from build123d import *
from OCP.BRepFilletAPI import BRepFilletAPI_MakeChamfer

# Parameters (mm, degrees)
SKETCH1_W               = 120
SKETCH1_H               = 38
SKETCH1_W_2             = 41
SKETCH1_H_2             = 21
BOSS_EXTRUDE1_DEPTH     = 11
SKETCH2_R               = 1.3
CUT_EXTRUDE1_DEPTH      = 8
FILLET1_RADIUS          = 19
FILLET1_LENGTH          = 11
BOSS_EXTRUDE2_START     = 8
BOSS_EXTRUDE2_DEPTH     = 8
FILLET2_R               = 16
CUT_EXTRUDE2_DEPTH      = 66.741919656
CUT_EXTRUDE2_DEPTH_BACK = 66.741919656
BOSS_EXTRUDE3_START     = 8
BOSS_EXTRUDE3_OUTLINE_W = 32
BOSS_EXTRUDE3_OUTLINE_H = 8
BOSS_EXTRUDE3_DEPTH     = 49
SKETCH6_W               = 52
SKETCH6_H               = 38
BOSS_EXTRUDE4_DEPTH     = 8
CUT_EXTRUDE3_DEPTH      = 74.518705262
CUT_EXTRUDE3_DEPTH_BACK = 74.518705262
SKETCH7_W               = 31
SKETCH7_H               = 13
SKETCH8_W               = 13
SKETCH8_H               = 23
CUT_EXTRUDE4_DEPTH      = 8
BOSS_EXTRUDE5_START     = -2
SKETCH9_R               = 9
BOSS_EXTRUDE5_DEPTH     = 2
SKETCH10_R              = 6.5
CUT_EXTRUDE5_DEPTH      = 8
SKETCH12_W              = 5
SKETCH12_H              = 6
CUT_EXTRUDE6_DEPTH      = 20
CHAMFER1_SIZE           = 6
CHAMFER1_SIZE_2         = 20
FILLET3_R               = 8
FILLET4_R               = 6
FILLET5_R               = 6
FILLET6_R               = 2.5
SKETCH13_R              = 1.1
CUT_EXTRUDE7_DEPTH      = 8
CUT_EXTRUDE8_DEPTH      = 69.483574828
CUT_EXTRUDE8_DEPTH_BACK = 69.483574828
CUT_EXTRUDE9_DEPTH      = 66.741919805
CUT_EXTRUDE9_DEPTH_BACK = 66.741919805
SKETCH15_R              = 1.3
SKETCH16_R              = 1.1
BOSS_EXTRUDE6_DEPTH     = 8
SKETCH17_R              = 1
CUT_EXTRUDE10_DEPTH     = 7


# Read off the part's stored shape, not the designer's step: Boss-Extrude3
# Some blends are built 0.0001 mm under size
with BuildPart() as part:
    # Sketch1 → Boss-Extrude1 (new body)
    with BuildSketch(Plane.XY):
        Rectangle(SKETCH1_W, SKETCH1_H)
        with Locations((-24.5, 0)):
            Rectangle(SKETCH1_W_2, SKETCH1_H_2, mode=Mode.SUBTRACT)
    extrude(amount=BOSS_EXTRUDE1_DEPTH)

    # Sketch2 → Cut-Extrude1 (cut)
    with BuildSketch(Plane.XY.offset(1)):
        with Locations((0, 5)):
            Circle(SKETCH2_R)
        with Locations((-48, 5)):
            Circle(SKETCH2_R)
        with Locations((-48, -5)):
            Circle(SKETCH2_R)
        with Locations((0, -5)):
            Circle(SKETCH2_R)
    extrude(amount=CUT_EXTRUDE1_DEPTH, mode=Mode.SUBTRACT)

    # Fillet1: full round fillet: the end face becomes a half cylinder, R = half its width
    fillet1_face = Plane((-60, 0, 5.5), x_dir=(0, 0, 1), z_dir=(-1, 0, 0))  # on the end face: x along it, z out of the body
    fillet1_slab = fillet1_face.offset(-FILLET1_RADIUS / 2) * Box(FILLET1_LENGTH, 2 * FILLET1_RADIUS, FILLET1_RADIUS, mode=Mode.PRIVATE)  # the body's end, R deep
    fillet1_round = Plane((-41, 0, 5.5), x_dir=(-1, 0, 0), z_dir=(0, 0, 1)) * Cylinder(FILLET1_RADIUS, FILLET1_LENGTH, mode=Mode.PRIVATE)  # its axis R under the face
    add(fillet1_slab - fillet1_round, mode=Mode.SUBTRACT)

    # Sketch3 → Boss-Extrude2 (add)
    with BuildSketch(Plane.XY.offset(11).offset(BOSS_EXTRUDE2_START)):
        with BuildLine():
            Line((60, 19), (-41, 19))
            ThreePointArc((-41, 19), (-60, 0), (-41, -19))
            Line((-41, -19), (60, -19))
            Line((60, -19), (60, 19))
        make_face()
        with BuildLine():
            Line((57, 16), (-41, 16))
            ThreePointArc((-41, 16), (-57, 0), (-41, -16))
            Line((-41, -16), (57, -16))
            Line((57, -16), (57, 16))
        make_face(mode=Mode.SUBTRACT)
    extrude(amount=-BOSS_EXTRUDE2_DEPTH)

    # Fillet2
    fillet2_edges = [part.edges().sort_by_distance(p)[0] for p in [
        (57, 16, 15),
        (57, -16, 15),
    ]]
    fillet(fillet2_edges, radius=FILLET2_R - 0.0001)  # a hair under: the kernel refuses the full size

    # Sketch4 → Cut-Extrude2 (cut, two sides: drawn at the far end of the back side and taken through both)
    with BuildSketch(Plane(origin=(0, 0, 0), x_dir=(1, 0, 0), z_dir=(0, 1, 0)).offset(-CUT_EXTRUDE2_DEPTH_BACK)):
        with BuildLine():
            Line((-60, -13.67), (-60, -19))
            Line((-60, -19), (-20, -19))
            add(Edge.make_bspline(
                [(-60, -13.67), (-53.560147586, -13.588290525), (-48.332037755, -13.416667168), (-40.159488654, -14.861068215), (-37.804599967, -16.297682364), (-29.745918458, -18.344163696), (-24.82962643, -18.478671578), (-20, -19)],
                knots=[0, 0, 0, 0, 0.436512255, 0.505229669, 0.666958087, 0.718456725, 1, 1, 1, 1], degree=3))
        make_face()
    extrude(amount=CUT_EXTRUDE2_DEPTH + CUT_EXTRUDE2_DEPTH_BACK, mode=Mode.SUBTRACT)

    # Boss-Extrude3 outline → Boss-Extrude3 (add)
    with BuildSketch(Plane.YZ.offset(BOSS_EXTRUDE3_START)):
        with Locations((0, 15)):
            Rectangle(BOSS_EXTRUDE3_OUTLINE_W, BOSS_EXTRUDE3_OUTLINE_H)
    extrude(amount=BOSS_EXTRUDE3_DEPTH)

    # Sketch6 → Boss-Extrude4 (add)
    with BuildSketch(Plane(origin=(0, 0, 0), x_dir=(-1, 0, 0), z_dir=(0, 0, -1))):
        with Locations((-34, 0)):
            Rectangle(SKETCH6_W, SKETCH6_H)
    extrude(amount=BOSS_EXTRUDE4_DEPTH)

    # Sketch7 → Cut-Extrude3 (cut, two sides: drawn at the far end of the back side and taken through both)
    with BuildSketch(Plane(origin=(0, 19, 0), x_dir=(1, 0, 0), z_dir=(0, 1, 0)).offset(-CUT_EXTRUDE3_DEPTH_BACK)):
        with Locations((34.5, -5.5)):
            Rectangle(SKETCH7_W, SKETCH7_H)
    extrude(amount=CUT_EXTRUDE3_DEPTH + CUT_EXTRUDE3_DEPTH_BACK, mode=Mode.SUBTRACT)

    # Sketch8 → Cut-Extrude4 (cut)
    with BuildSketch(Plane.ZY.offset(-50)):
        with Locations((5.5, 0)):
            Rectangle(SKETCH8_W, SKETCH8_H)
    extrude(amount=-CUT_EXTRUDE4_DEPTH, mode=Mode.SUBTRACT)

    # Sketch9 → Boss-Extrude5 (add)
    with BuildSketch(Plane(origin=(0, 0, 0), x_dir=(-1, 0, 0), z_dir=(0, 0, -1)).offset(BOSS_EXTRUDE5_START)):
        with BuildLine():
            Line((-8, 19), (-8, -19))
            Line((-8, -19), (41, -19))
            ThreePointArc((41, -19), (60, 0), (41, 19))
            Line((41, 19), (-8, 19))
        make_face()
        with Locations((34.75, 0)):
            Circle(SKETCH9_R, mode=Mode.SUBTRACT)
    extrude(amount=BOSS_EXTRUDE5_DEPTH)

    # Sketch10 → Cut-Extrude5 (cut)
    with BuildSketch(Plane(origin=(60, 0, 0), x_dir=(0, 0, -1), z_dir=(1, 0, 0))):
        with Locations(Location((-5.5, 5.3, 0), (0, 0, 90))):
            Circle(SKETCH10_R)
    extrude(amount=-CUT_EXTRUDE5_DEPTH, mode=Mode.SUBTRACT)

    # Sketch12 → Cut-Extrude6 (cut)
    with BuildSketch(Plane(origin=(19, 0, 0), x_dir=(0, 0, -1), z_dir=(1, 0, 0))):
        with Locations((-5.5, 16)):
            Rectangle(SKETCH12_W, SKETCH12_H)
        with Locations((-5.5, -16)):
            Rectangle(SKETCH12_W, SKETCH12_H)
    extrude(amount=-CUT_EXTRUDE6_DEPTH, mode=Mode.SUBTRACT)

    # Chamfer1
    chamfer1_edges_1 = [part.edges().sort_by_distance(p)[0] for p in [
        (-1, -13, 5.5),
    ]]
    chamfer1_side_1 = [part.faces().sort_by_distance(p)[0] for p in [
        (-1, -13.12, 5.5),
    ]]
    chamfer1_edges_2 = [part.edges().sort_by_distance(p)[0] for p in [
        (-1, 13, 5.5),
    ]]
    chamfer1_side_2 = [part.faces().sort_by_distance(p)[0] for p in [
        (-1, 13.12, 5.5),
    ]]
    chamfer1 = BRepFilletAPI_MakeChamfer(part.part.solid().wrapped)
    for e in chamfer1_edges_1:
        chamfer1.Add(CHAMFER1_SIZE - 0.0001, CHAMFER1_SIZE_2 - 0.0001, e.wrapped, chamfer1_side_1[0].wrapped)
    for e in chamfer1_edges_2:
        chamfer1.Add(CHAMFER1_SIZE - 0.0001, CHAMFER1_SIZE_2 - 0.0001, e.wrapped, chamfer1_side_2[0].wrapped)
    add(Compound.cast(chamfer1.Shape()), mode=Mode.REPLACE)  # a hair under: the kernel refuses the full size

    # Fillet3
    # the kernel refuses this fillet: 8 mm, written as the material it takes off along each edge
    with BuildSketch(Plane(origin=(19, 19, -1), x_dir=(0, -1, 0), z_dir=(0, 0, 1))) as fillet3_piece_1_section:
        with BuildLine():
            CenterArc((FILLET3_R, -FILLET3_R), FILLET3_R, 90, 90)
            Line((0, -FILLET3_R), (0, 0))
            Line((0, 0), (FILLET3_R, 0))
        make_face()
    fillet3_piece_1 = extrude(amount=24, mode=Mode.PRIVATE)
    fillet3_piece_1 = split(fillet3_piece_1, bisect_by=Plane(origin=(18.924002019, 12.501601439, 12), z_dir=(0, 0, -1)), keep=Keep.TOP, mode=Mode.PRIVATE)
    add(fillet3_piece_1, mode=Mode.SUBTRACT)
    with BuildSketch(Plane(origin=(19, -19, 23), x_dir=(0, 1, 0), z_dir=(0, 0, -1))) as fillet3_piece_2_section:
        with BuildLine():
            CenterArc((FILLET3_R, -FILLET3_R), FILLET3_R, 90, 90)
            Line((0, -FILLET3_R), (0, 0))
            Line((0, 0), (FILLET3_R, 0))
        make_face()
    fillet3_piece_2 = extrude(amount=24, mode=Mode.PRIVATE)
    fillet3_piece_2 = split(fillet3_piece_2, bisect_by=Plane(origin=(18.924002019, -12.501601439, 12), z_dir=(0, 0, -1)), keep=Keep.TOP, mode=Mode.PRIVATE)
    add(fillet3_piece_2, mode=Mode.SUBTRACT)

    # Fillet4
    # the kernel refuses this fillet: 6 mm, written as the material it takes off along each edge
    with BuildSketch(Plane(origin=(-28, -19, -8), x_dir=(0, 0, 1), z_dir=(1, 0, 0)), Plane(origin=(96, 19, -8), x_dir=(0, 0, 1), z_dir=(-1, 0, 0))) as fillet4_piece_1:
        with BuildLine():
            CenterArc((FILLET4_R, -FILLET4_R), FILLET4_R, 90, 90)
            Line((0, -FILLET4_R), (-FILLET4_R * 0.02, -FILLET4_R))
            Line((-FILLET4_R * 0.02, -FILLET4_R), (-FILLET4_R * 0.02, FILLET4_R * 0.02))
            Line((-FILLET4_R * 0.02, FILLET4_R * 0.02), (FILLET4_R, FILLET4_R * 0.02))
            Line((FILLET4_R, FILLET4_R * 0.02), (FILLET4_R, 0))
        make_face()
    extrude(amount=124, mode=Mode.SUBTRACT)
    with BuildSketch(Plane(origin=(96, 19, 19), x_dir=(0, 0, -1), z_dir=(-1, 0, 0)), Plane(origin=(-56, -19, 19), x_dir=(0, 0, -1), z_dir=(1, 0, 0))) as fillet4_piece_2:
        with BuildLine():
            CenterArc((FILLET4_R, FILLET4_R), FILLET4_R, 180, 90)
            Line((0, FILLET4_R), (-FILLET4_R * 0.02, FILLET4_R))
            Line((-FILLET4_R * 0.02, FILLET4_R), (-FILLET4_R * 0.02, -FILLET4_R * 0.02))
            Line((-FILLET4_R * 0.02, -FILLET4_R * 0.02), (FILLET4_R, -FILLET4_R * 0.02))
            Line((FILLET4_R, -FILLET4_R * 0.02), (FILLET4_R, 0))
        make_face()
    extrude(amount=152, mode=Mode.SUBTRACT)

    # Fillet5
    fillet5_edges = [part.edges().sort_by_distance(p)[0] for p in [
        (8, 0, 0),
    ]]
    fillet(fillet5_edges, radius=FILLET5_R)

    # Fillet6
    fillet6_edges = [part.edges().sort_by_distance(p)[0] for p in [
        (8.862066808, 16.041314475, 3),
        (8.862066808, 16.041314475, 8),
        (8.862066808, -16.041314475, 8),
        (8.862066808, -16.041314475, 3),
    ]]
    fillet(fillet6_edges, radius=FILLET6_R - 0.0001)  # a hair under: the kernel refuses the full size

    # Sketch13 → Cut-Extrude7 (cut)
    with BuildSketch(Plane.ZY.offset(-50)):
        with Locations((6.5, 13.8)):
            Circle(SKETCH13_R)
        with Locations((6.5, -13.8)):
            Circle(SKETCH13_R)
    extrude(amount=-CUT_EXTRUDE7_DEPTH, mode=Mode.SUBTRACT)

    # Sketch14 → Cut-Extrude8 (cut, two sides: drawn at the far end of the back side and taken through both)
    with BuildSketch(Plane.XY.offset(19).offset(-CUT_EXTRUDE8_DEPTH_BACK)):
        Polygon((5, 19), (60, 16.5), (60, 19), align=None)
        Polygon((60, -19), (60, -16.5), (5, -19), align=None)
    extrude(amount=CUT_EXTRUDE8_DEPTH + CUT_EXTRUDE8_DEPTH_BACK, mode=Mode.SUBTRACT)

    # Sketch15 → Cut-Extrude9 (cut, two sides: drawn at the far end of the back side and taken through both)
    with BuildSketch(Plane.XY.offset(11).offset(-CUT_EXTRUDE9_DEPTH_BACK)):
        with Locations((0, -5)):
            Circle(SKETCH15_R)
        with Locations((-48, -5)):
            Circle(SKETCH15_R)
        with Locations((-48, 5)):
            Circle(SKETCH15_R)
        with Locations((0, 5)):
            Circle(SKETCH15_R)
    extrude(amount=CUT_EXTRUDE9_DEPTH + CUT_EXTRUDE9_DEPTH_BACK, mode=Mode.SUBTRACT)

    # Sketch16 → Boss-Extrude6 (add)
    with BuildSketch(Plane.ZY.offset(-50)):
        with Locations((6.5, -13.8)):
            Circle(SKETCH16_R)
        with Locations((6.5, 13.8)):
            Circle(SKETCH16_R)
    extrude(amount=-BOSS_EXTRUDE6_DEPTH)

    # Sketch17 → Cut-Extrude10 (cut)
    with BuildSketch(Plane.ZY.offset(-50)):
        with Locations((5.5, -13.6)):
            Circle(SKETCH17_R)
        with Locations((5.5, 14)):
            Circle(SKETCH17_R)
    extrude(amount=-CUT_EXTRUDE10_DEPTH, mode=Mode.SUBTRACT)


solid = part.part
Can you work these out from the model? Positions are in its coordinate system, mm. A direction names the side the tool comes from. Coordinates: 2 decimals unless noted, no trailing zeros. Write each question's results on one line, items separated by ' | '. Start each with the question number.
Q1. If I drill on probe 1 along Y at (x, z) = (-13.5, 3.5); probe 2 along Z at (x, y) = (22, 6.5); probe 3 along Y at (x, z) = (-34.75, 0.7), over which ranges is the centre line in solid material (lowest first)?
Q2. Imagine slicing it at A-A (x = -48). State how many separate pieces and enclosed holes the cut face has, then the cut area to 3 significant figures.
Q3. I'm going to push flat-ended pins straight in: pin 1 (1.8 mm diameter, centred on y = -13.6, z = 5.5, fed in from -X); pin 2 (1 mm diameter, centred on x = 14, z = 14, fed in from +Y); pin 3 (6 mm diameter, centred on x = -41, y = 9.5, fed in from -Z). Where does each tip first touch, or does it pass through?
Q4. We'd pull the mould along X, two halves only. Please class faces 1 (the face through (38.996, -17.455, -2.922)), 2 (the face through (-20, 0, 2)), 3 (the face through (-60, 0, 7)), 4 (the face through (-49.3, -4.94, 5.42)): +X half, -X half, draft (parallel to the pull), parting line (faces both ways), or undercut.
Q5. On a 3-axis mill with a long thin cutter (end or side, diameter ignored), from which of +Z, -Z, +X, -X, +Y, -Y can I reach the whole of each face in a straight line? I mean faces 5 (the face through (54, -11.5, 5)), 6 (the face through (-25, -10.5, 6)), 7 (the face through (58.093, 11.744, 4.651)), 8 (the face through (9.13, -16.45, 4.04)), 9 (the face through (9.13, 16.45, 6.96)). Say none if no direction works.
Taken from the geometry:
1) probe 1: y = -19 to -10.5, 10.5 to 19 | probe 2: z = -8 to -1, 12 to 19 | probe 3: y = -19 to -9, 9 to 19
2) separate pieces: 3 | enclosed holes: 0 | area: 350 mm^2
3) pin 1: stops at x = -55.13 | pin 2: stops at y = 18.61 | pin 3: stops at z = 0
4) face 1: +X half | face 2: undercut | face 3: -X half | face 4: undercut
5) face 5: none | face 6: +Z | face 7: +X | face 8: -Y | face 9: +Y
